Can you work these out from the model? Positions are in its coordinate system, mm. A direction names the side the tool comes from. Round coordinates to 2 decimals unless told otherwise and drop trailing zeros. Loops run counter-clockwise (first coordinate to the right, second up) from the corner with the lowest first, then second, coordinate; pieces in that order, holes last. Notation, with made-up numbers: M 76.5,-31 L 118.5,-31 A16 ccw 118.5,-22 Z; hole C -4,-15 d10. An arc over 180 degrees is marked long. Return JSON: item names as keys, results as strings.
```python
from build123d import *

# Parameters (mm, degrees)
SKETCH1_W               = 127
SKETCH1_H               = 127
BOSS_EXTRUDE1_DEPTH     = 4.7625
SKETCH2_W               = 3.175
SKETCH2_H               = 127
BOSS_EXTRUDE2_DEPTH     = 88.9
SKETCH3_R               = 6.35
CUT_EXTRUDE1_DEPTH      = 48.244
CUT_EXTRUDE1_DEPTH_BACK = 80.756
FILLET1_R               = 3.175
CHAMFER1_SIZE           = 25.4
CUT_EXTRUDE4_START      = -5.7625
SKETCH4_R               = 3.175
CUT_EXTRUDE4_DEPTH      = 95.6625
FILLET5_R               = 12.7
CUT_EXTRUDE5_DEPTH      = 48.244
CUT_EXTRUDE5_DEPTH_BACK = 80.756


with BuildPart() as part:
    # Sketch1 → Boss-Extrude1 (new body)
    with BuildSketch(Plane(origin=(0, 0, 0), x_dir=(1, 0, 0), z_dir=(0, 1, 0))):
        Rectangle(SKETCH1_W, SKETCH1_H)
    extrude(amount=BOSS_EXTRUDE1_DEPTH)

    # Sketch2 → Boss-Extrude2 (add)
    with BuildSketch(Plane(origin=(0, 4.7625, 0), x_dir=(1, 0, 0), z_dir=(0, 1, 0))):
        with Locations((-14.6685, 0)):
            Rectangle(SKETCH2_W, SKETCH2_H)
        with Locations((14.6685, 0)):
            Rectangle(SKETCH2_W, SKETCH2_H)
    extrude(amount=BOSS_EXTRUDE2_DEPTH)

    # Sketch3 → Cut-Extrude1 (cut, two sides)
    with BuildSketch(Plane.ZY.offset(16.256)) as cut_extrude1_sk:
        with Locations((0, 61.9125)):
            Circle(SKETCH3_R)
    extrude(amount=CUT_EXTRUDE1_DEPTH, mode=Mode.SUBTRACT)
    extrude(cut_extrude1_sk.sketch, amount=-CUT_EXTRUDE1_DEPTH_BACK, mode=Mode.SUBTRACT)

    # Fillet1
    fillet1_edges = [part.edges().sort_by_distance(p)[0] for p in [
        (-16.256, 4.7625, 0),
        (-13.081, 4.7625, 0),
        (13.081, 4.7625, 0),
        (16.256, 4.7625, 0),
    ]]
    fillet(fillet1_edges, radius=FILLET1_R)

    # Chamfer1
    chamfer1_edges = [part.edges().sort_by_distance(p)[0] for p in [
        (-14.6685, 93.6625, 63.5),
        (-14.6685, 93.6625, -63.5),
        (14.6685, 93.6625, 63.5),
        (14.6685, 93.6625, -63.5),
    ]]
    chamfer(chamfer1_edges, length=CHAMFER1_SIZE)

    # Sketch4 → Cut-Extrude4 (cut)
    with BuildSketch(Plane(origin=(0, 4.7625, 0), x_dir=(1, 0, 0), z_dir=(0, 1, 0)).offset(CUT_EXTRUDE4_START)):
        with Locations((-50.8, -50.8)):
            Circle(SKETCH4_R)
        with Locations((-50.8, 50.8)):
            Circle(SKETCH4_R)
    cut_extrude4 = extrude(amount=CUT_EXTRUDE4_DEPTH, mode=Mode.SUBTRACT)

    # Mirror2: Cut-Extrude4 across plane
    add(cut_extrude4.mirror(Plane.ZY), mode=Mode.SUBTRACT)

    # Fillet5
    fillet5_edges = [part.edges().sort_by_distance(p)[0] for p in [
        (-63.5, 2.38125, -63.5),
        (63.5, 2.38125, -63.5),
        (63.5, 2.38125, 63.5),
        (-63.5, 2.38125, 63.5),
    ]]
    fillet(fillet5_edges, radius=FILLET5_R)

    # Sketch7 → Cut-Extrude5 (cut, two sides)
    with BuildSketch(Plane.ZY.offset(16.256)) as cut_extrude5_sk:
        Polygon((-63.5, 36.5125), (-14.62430355, 93.6625), (-38.1, 93.6625), (-63.5, 68.2625), align=None)
        Polygon((38.1, 93.6625), (14.62430355, 93.6625), (63.5, 36.5125), (63.5, 68.2625), align=None)
    extrude(amount=CUT_EXTRUDE5_DEPTH, mode=Mode.SUBTRACT)
    extrude(cut_extrude5_sk.sketch, amount=-CUT_EXTRUDE5_DEPTH_BACK, mode=Mode.SUBTRACT)


solid = part.part
```
Q1. On a 3-axis mill with a long thin cutter (end or side, diameter ignored), from which of +Z, -Z, +X, -X, +Y, -Y can I reach the whole of each face in a straight line? I mean faces 5 (the flat face through (-0.2, 4.6, -63.5)), 6 (the cylindrical face through (12.13, 5.67, -0.89)), 7 (the flat face through (-42, 4.762, -1)). Say none if no direction works.
Results:
{"face 5": "-Z, +X, -X, +Y, -Y", "face 6": "+Z, -Z, +Y", "face 7": "+Z, -Z, -X, +Y"}
Q2. Suppose I cut it at B-B, the plane y = 86.5. Please give me the cut outline in (x, z), plus the area to 3 significant figures.
Results:
{"outline": "M -16.26,-20.75 L -13.08,-20.75 L -13.08,20.75 L -16.26,20.75 Z; M 13.08,-20.75 L 16.26,-20.75 L 16.26,20.75 L 13.08,20.75 Z", "area": "264 mm2"}
Q3. Thinking about a two-plate mould opening in Z: for faces 1 (the cylindrical face through (-51.21, 2.35, -53.95)), 2 (the flat face through (13.081, 41, 1)), 3 (the cylindrical face through (59.88, 2.41, -59.68)), 4 (the flat face through (-0.2, 4.6, 63.5)), which applies, pulls with the +Z half, pulls with the -Z half, needs draft (parallel to the pull), parting line crosses it, or undercut?
Results:
{"face 1": "undercut", "face 2": "needs draft", "face 3": "pulls with the -Z half", "face 4": "pulls with the +Z half"}
Q4. I'm going to push flat-ended pins straight in: pin 1 Ø12 at (y, z) = (65.5, -13.5) entering from -X; pin 2 Ø5 at (y, z) = (77.5, 5.5) entering from +X; pin 3 Ø16 at (x, z) = (-4, 31.5) entering from +Y; pin 4 Ø4 at (x, z) = (50.8, -50.8) entering from +Y. Where does each tip first touch, or does it pass through?
Results:
{"pin 1": "stops at x = -16.26", "pin 2": "stops at x = 16.26", "pin 3": "stops at y = 5.55", "pin 4": "passes through"}
Q5. Suppose I cut it at A-A, the plane z = 0. State how many separate pieces and enclosed holes the cut face has, plus the area to 3 significant figures.
Results:
{"separate pieces": "3", "enclosed holes": "0", "area": "1,100 mm2"}
Q6. Suppose I cut it at D-D, the plane y = 40. Please give me the cut outline in (x, z), plus the area to 3 significant figures.
Results:
{"outline": "M -16.26,-60.52 L -13.08,-60.52 L -13.08,60.52 L -16.26,60.52 Z; M 13.08,-60.52 L 16.26,-60.52 L 16.26,60.52 L 13.08,60.52 Z", "area": "769 mm2"}
Q7. If I drill on line 1 along Z through (x, y) = (-50.8, 2.6) (3 decimals); line 2 along X through (y, z) = (28, 50); line 3 along X through (y, z) = (1, 50), over which ranges is the centre line in solid material (lowest first)?
Results:
{"line 1": "z = -63.5 to -53.975, -47.625 to 47.625, 53.975 to 63.5", "line 2": "x = -16.26 to -13.08, 13.08 to 16.26", "line 3": "x = -63.5 to -53.87, -47.73 to 47.73, 53.87 to 63.5"}
